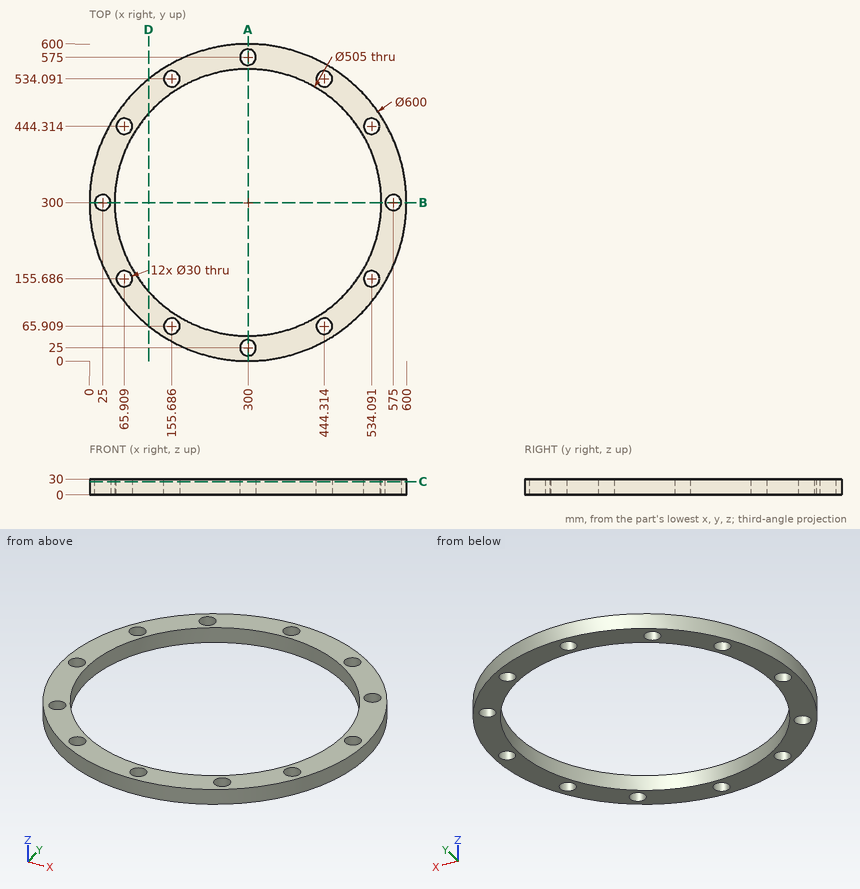
Verification items for this drawing (mm, ordinates from the low corner). Coordinates: 2 decimals unless noted, no trailing zeros. Order: outer loops, then holes, each group sorted by start corner. A loop starts at its lowest first (then second) coordinate and runs counter-clockwise, first axis right, second up.
Q1. Thickness scan on probe 1 along X at (y, z) = (455, 29) (1 decimal); probe 2 along Y at (x, z) = (451, 16.25) (1 decimal); probe 3 along Y at (x, z) = (564, 25). Record the ranges inside material, lowest first.
Reply:
probe 1: x = 43.1 to 55.4, 76.4 to 100.7, 499.3 to 523.6, 544.6 to 556.9
probe 2: y = 40.8 to 52.5, 79.3 to 97.6, 502.4 to 520.7, 547.5 to 559.2
probe 3: y = 157.51 to 289.8, 310.2 to 442.49
Q2. Sectioned sample at A-A on x = 300. Record the cut outline in (y, z).
Reply:
outline: (0, 0) - (10, 0) - (10, 30) - (0, 30) - close; (40, 0) - (47.5, 0) - (47.5, 30) - (40, 30) - close; (552.5, 0) - (560, 0) - (560, 30) - (552.5, 30) - close; (590, 0) - (600, 0) - (600, 30) - (590, 30) - close
Q3. Depth check by flat-ended pin: pin 1 Ø4 at (y, z) = (522.5, 19.5) entering from +X; pin 2 Ø8 at (x, z) = (220.5, 9) entering from +Y; pin 3 Ø1 at (x, z) = (211.5, 19.5) entering from -Y; pin 4 Ø18 at (x, y) = (534.09, 444.31) entering from -Z. Enter the tip coordinate at first touch or a pass-through.
Reply:
pin 1: stops at x = 503.42
pin 2: stops at y = 590.34
pin 3: stops at y = 13.2
pin 4: passes through
Q4. Sectioned sample at C-C on z = 25. Give the number of separate pieces and of enclosed holes in the cut face, and give its area (3 significant figures).
Reply:
separate pieces: 1
enclosed holes: 13
area: 74,000 mm2
Q5. Sectioned sample at D-D on x = 112. Record the cut outline in (y, z).
Reply:
outline: (66.21, 0) - (131.44, 0) - (131.44, 30) - (66.21, 30) - close; (468.56, 0) - (533.79, 0) - (533.79, 30) - (468.56, 30) - close
